Can you work these out from the model? Positions are in its coordinate system, mm. A direction names the side the tool comes from. Give positions to 0.01 mm unless a question says otherwise; leave off trailing zeros. Write each loop counter-clockwise with the first axis right and the second up, starting at its lowest first coordinate (ties: lowest second). Pieces come first, ordered by that corner, then holes. Notation, with made-up numbers: (62, 7.5) -> (100, 7.5) arc R15 cw to (100, 27.5) -> close; hole circle Ø6 at (-32.75, 33). An arc over 180 degrees is marked (long way). One line per item, written item: value.
from build123d import *

# Parameters (mm, degrees)
F0_R        = 25
F1_DEPTH    = 20
F3_DEPTH    = 70
F4_R        = 5
F6_DEPTH    = 25
F7_T1_DEPTH = 17.5
F7_T3_DEPTH = 30
F8_R        = 4.99999


# Not quite as in the source:
# - a fillet or chamfer that OpenCascade refuses, or shapes differently, is made with other operations: its cross-section is extruded or revolved along the edge and cut away or added
# - a fillet or chamfer is up to 0.001 mm smaller than in the source, because OpenCascade refuses the exact size


with BuildPart() as f1:
    # F0 (on Front) → F1 (new body)
    with BuildSketch(Plane.XZ):
        with BuildLine():
            Line((-25.1910626888, 440.0464960357), (-25.1910626888, -86.4124843018))
            Line((-25.1910626888, -86.4124843018), (24.8089373112, -86.4124843018))
            Line((24.8089373112, -86.4124843018), (24.8089373112, 440.0464960357))
            ThreePointArc((24.8089373112, 440.0464960357), (25.5893928539, 443.9194793819), (27.8089373112, 447.1879244642))
            ThreePointArc((27.8089373112, 447.1879244642), (-0.1910626888, 515.7536381784), (-28.1910626888, 447.1879244642))
            ThreePointArc((-28.1910626888, 447.1879244642), (-25.9715182315, 443.9194793819), (-25.1910626888, 440.0464960357))
        make_face()
        with Locations((-0.1910626888, 475.7536381784)):
            Circle(F0_R, mode=Mode.SUBTRACT)
    extrude(amount=F1_DEPTH)

    # F2 (on face) → F3 (cut, symmetric)
    with BuildSketch(Plane(origin=(-25.1910626888, 0, 0), x_dir=(0, -1, 0), z_dir=(-1, 0, 0))):
        Polygon((12.5, 447.1879244642), (12.5, 450.7536381784), (12.5, 515.7536381784), (7.5, 515.7536381784), (7.5, 450.7536381784), (7.5, 447.1879244642), (7.5, 443.61721025), (12.5, 443.61721025), align=None)
    extrude(amount=F3_DEPTH, both=True, mode=Mode.SUBTRACT)

    # F4
    f4_edges = [f1.edges().sort_by_distance(p)[0] for p in [
        (-25.191063, -20, 176.817006),
        (-25.191063, 0, 176.817006),
    ]]
    fillet(f4_edges, radius=F4_R)

    # F5 (on Right) → F6 (join, symmetric)
    with BuildSketch(Plane.YZ):
        Polygon((0, -91.4124843018), (0, -86.4124843018), (-20, -86.4124843018), (-100, -86.4124843018), (-100, -91.4124843018), align=None)
    extrude(amount=F6_DEPTH, both=True)

    # F7: fillet of radius 5 on 4 edges, made by hand

    # F7_s2 → F7_t1 (cut)
    with BuildSketch(Plane.XY.offset(-103.9124843018)):
        with BuildLine():
            ThreePointArc((-20, 0), (-23.5355339059, -1.4644660941), (-25, -5))
            Line((-25, -5), (-25, 0))
            Line((-25, 0), (-20, 0))
        make_face()
    extrude(amount=F7_T1_DEPTH, mode=Mode.SUBTRACT)

    # F7_s4 → F7_t3 (cut)
    with BuildSketch(Plane.XY.offset(-103.9124843018)):
        with BuildLine():
            ThreePointArc((20, 0), (23.5355339059, -1.4644660941), (25, -5))
            Line((25, -5), (25, 0))
            Line((25, 0), (20, 0))
        make_face()
        with BuildLine():
            ThreePointArc((-20, -100), (-23.5355339059, -98.5355339059), (-25, -95))
            Line((-25, -95), (-25, -100))
            Line((-25, -100), (-20, -100))
        make_face()
        with BuildLine():
            ThreePointArc((25, -95), (23.5355339059, -98.5355339059), (20, -100))
            Line((20, -100), (25, -100))
            Line((25, -100), (25, -95))
        make_face()
    extrude(amount=F7_T3_DEPTH, mode=Mode.SUBTRACT)

    # F8 (radius 5 in the source; OpenCascade refuses exactly that, so slightly less here)
    f8_edges = [f1.edges().sort_by_distance(p)[0] for p in [
        (23.535534, -98.535534, -91.412484),
        (25, -50, -91.412484),
        (23.535534, -1.464466, -91.412484),
        (0, 0, -91.412484),
        (-23.535534, -1.464466, -91.412484),
        (-25, -50, -91.412484),
        (-23.535534, -98.535534, -91.412484),
        (0, -100, -91.412484),
    ]]
    fillet(f8_edges, radius=F8_R)


solid = f1.part
1) Will these pins go through, and if not, where does the flat tip stop? pin 1 (25 mm diameter, centred on x = -7.5, y = -44.5, fed in from +Z); pin 2 (5.5 mm diameter, centred on x = -23.5, y = -11.5, fed in from -Z); pin 3 (8 mm diameter, centred on x = 27.5, z = 86, fed in from -Y).
Answer list:
pin 1: stops at z = -86.41
pin 2: stops at z = -91.36
pin 3: stops at y = -18.37
2) For faces 5 (the face through (-25.191, -10, 181)), 6 (the face through (-19, -7.5, 496)), 7 (the face through (-1, -20, 216)), which set-ups out of +Z, -Z, +X, -X, +Y, -Y let a thin tool reach every point of the face, with its end or its side?
Answer list:
face 5: -Z, -X, +Y, -Y
face 6: +Z, +X, -X
face 7: +Z, +X, -X, -Y
3) If we section it at A-A (z = 402): Write out the boundary of the cut face in (x, y).
Answer list:
outline: (-25.19, -15) arc R5 ccw to (-20.19, -20) -> (19.81, -20) arc R5 ccw to (24.81, -15) -> (24.81, -5) arc R5 ccw to (19.81, 0) -> (-20.19, 0) arc R5 ccw to (-25.19, -5) -> close
4) We'd pull the mould along Z, two halves only. Please class faces 1 (the face through (0, 0, 208)), 2 (the face through (1.13, -6.23, 515.73)), 3 (the face through (0, -51, -91.412)), 4 (the face through (-3.45, -3.7, 500.54)): released by +Z, released by -Z, zero draft, split by the parting line, or undercut.
Answer list:
face 1: zero draft
face 2: split by the parting line
face 3: released by -Z
face 4: undercut
5) I need wall thicknesses on L1, parallel to Y at x = -20.5, z = 432; L2, parallel to X at y = -11.5, z = -0.5; L3, parallel to Z at x = 12, y = -70.5. Which ranges of each line are inside material? Lowest first, please.
Answer list:
L1: y = -19.99 to -0.01
L2: x = -25.19 to 24.81
L3: z = -91.41 to -86.41
6) If we section it at C-C (x = 14.5): State how many separate pieces and enclosed holes the cut face has, and give its area (3 significant figures).
Answer list:
separate pieces: 3
enclosed holes: 0
area: 11,500 mm^2
